Build history of the part. All positions in model axes, mm. A direction names the side the tool comes from. Round coordinates to 2 decimals unless told otherwise and drop trailing zeros. Loops run counter-clockwise (first coordinate to the right, second up) from the corner with the lowest first, then second, coordinate; pieces in that order, holes last.
from build123d import *

# Parameters (mm, degrees)
SKETCH1_R                    = 33.334829616
SKETCH1_R_2                  = 11
EXTRUDE1_DEPTH               = 10
SKETCH2_W                    = 68.7469374
SKETCH2_H                    = 68.7469374
CUT_EXTRUDE1_DEPTH           = 10
SKETCH3_R                    = 1.5
CUT_EXTRUDE2_DEPTH           = 32.563829392
SKETCH4_R                    = 2.25
CUT_EXTRUDE3_DEPTH           = 1.5
CUT_EXTRUDE3_DRAFT           = -28
CUT_EXTRUDE3_PROFILE_2_DEPTH = 1.5
CUT_EXTRUDE3_PROFILE_2_DRAFT = -28
CUT_EXTRUDE3_PROFILE_3_DEPTH = 1.5
CUT_EXTRUDE3_PROFILE_3_DRAFT = -28
CUT_EXTRUDE3_PROFILE_4_DEPTH = 1.5
CUT_EXTRUDE3_PROFILE_4_DRAFT = -28
SKETCH5_R                    = 13.5
CUT_EXTRUDE4_DEPTH           = 3


with BuildPart() as part:
    # Sketch1 → Extrude1 (new body)
    with BuildSketch(Plane(origin=(0, 0, 0), x_dir=(1, 0, 0), z_dir=(0, 1, 0))):
        with Locations(Location((0, 0, 0), (0, 0, 270))):
            Circle(SKETCH1_R)
        with Locations(Location((0, 0, 0), (0, 0, 270))):
            Circle(SKETCH1_R_2, mode=Mode.SUBTRACT)
    extrude(amount=EXTRUDE1_DEPTH)

    # Sketch2 → Cut-Extrude1 (cut)
    with BuildSketch(Plane.XZ):
        Rectangle(SKETCH2_W, SKETCH2_H)
        Polygon((16.16926222, 21.16926222), (21.16926222, 16.16926222), (21.16926222, -16.16926222), (16.16926222, -21.16926222), (-16.16926222, -21.16926222), (-21.16926222, -16.16926222), (-21.16926222, 16.16926222), (-16.16926222, 21.16926222), align=None, mode=Mode.SUBTRACT)
    extrude(amount=-CUT_EXTRUDE1_DEPTH, mode=Mode.SUBTRACT)

    # Sketch3 → Cut-Extrude2 (cut, through all)
    with BuildSketch(Plane(origin=(0, 10, 0), x_dir=(1, 0, 0), z_dir=(0, 1, 0))):
        with Locations(Location((-15.518439578, 15.481538459, 0), (0, 0, 270))):
            Circle(SKETCH3_R)
        with Locations(Location((-15.481538459, -15.518439578, 0), (0, 0, 270))):
            Circle(SKETCH3_R)
        with Locations(Location((15.481538459, 15.518439578, 0), (0, 0, 270))):
            Circle(SKETCH3_R)
        with Locations(Location((15.518439578, -15.481538459, 0), (0, 0, 270))):
            Circle(SKETCH3_R)
    extrude(amount=-CUT_EXTRUDE2_DEPTH, mode=Mode.SUBTRACT)


with BuildPart() as cut_extrude3_tool:
    # Sketch4 → Cut-Extrude3 (with draft: the straight prism first)
    with BuildSketch(Plane(origin=(0, 10, 0), x_dir=(1, 0, 0), z_dir=(0, 1, 0))):
        with Locations((-15.518439578, 15.481538459)):
            Circle(SKETCH4_R)
    extrude(amount=-CUT_EXTRUDE3_DEPTH)
    # Cut-Extrude3: the draft: its side faces are tilted about the plane it starts from
    cut_extrude3_sides = [cut_extrude3_tool.faces().sort_by_distance(p)[0] for p in [
        (-17.768439578, 9.25, -15.481538459),
    ]]
    draft(cut_extrude3_sides, Plane(origin=(0, 10, 0), x_dir=(1, 0, 0), z_dir=(0, 1, 0)), CUT_EXTRUDE3_DRAFT)


with BuildPart() as part_1:
    add(part.part)

    # Cut-Extrude3: cut by cut_extrude3_tool
    add(cut_extrude3_tool.part, mode=Mode.SUBTRACT)


with BuildPart() as cut_extrude3_profile_2_tool:
    # Sketch4 → Cut-Extrude3 profile 2 (with draft: the straight prism first)
    with BuildSketch(Plane(origin=(0, 10, 0), x_dir=(1, 0, 0), z_dir=(0, 1, 0))):
        with Locations((-15.481538459, -15.518439578)):
            Circle(SKETCH4_R)
    extrude(amount=-CUT_EXTRUDE3_PROFILE_2_DEPTH)
    # Cut-Extrude3 profile 2: the draft: its side faces are tilted about the plane it starts from
    cut_extrude3_profile_2_sides = [cut_extrude3_profile_2_tool.faces().sort_by_distance(p)[0] for p in [
        (-17.731538459, 9.25, 15.518439578),
    ]]
    draft(cut_extrude3_profile_2_sides, Plane(origin=(0, 10, 0), x_dir=(1, 0, 0), z_dir=(0, 1, 0)), CUT_EXTRUDE3_PROFILE_2_DRAFT)


with BuildPart() as part_2:
    add(part_1.part)

    # Cut-Extrude3 profile 2: cut by cut_extrude3_profile_2_tool
    add(cut_extrude3_profile_2_tool.part, mode=Mode.SUBTRACT)


with BuildPart() as cut_extrude3_profile_3_tool:
    # Sketch4 → Cut-Extrude3 profile 3 (with draft: the straight prism first)
    with BuildSketch(Plane(origin=(0, 10, 0), x_dir=(1, 0, 0), z_dir=(0, 1, 0))):
        with Locations((15.481538459, 15.518439578)):
            Circle(SKETCH4_R)
    extrude(amount=-CUT_EXTRUDE3_PROFILE_3_DEPTH)
    # Cut-Extrude3 profile 3: the draft: its side faces are tilted about the plane it starts from
    cut_extrude3_profile_3_sides = [cut_extrude3_profile_3_tool.faces().sort_by_distance(p)[0] for p in [
        (13.231538459, 9.25, -15.518439578),
    ]]
    draft(cut_extrude3_profile_3_sides, Plane(origin=(0, 10, 0), x_dir=(1, 0, 0), z_dir=(0, 1, 0)), CUT_EXTRUDE3_PROFILE_3_DRAFT)


with BuildPart() as part_3:
    add(part_2.part)

    # Cut-Extrude3 profile 3: cut by cut_extrude3_profile_3_tool
    add(cut_extrude3_profile_3_tool.part, mode=Mode.SUBTRACT)


with BuildPart() as cut_extrude3_profile_4_tool:
    # Sketch4 → Cut-Extrude3 profile 4 (with draft: the straight prism first)
    with BuildSketch(Plane(origin=(0, 10, 0), x_dir=(1, 0, 0), z_dir=(0, 1, 0))):
        with Locations((15.518439578, -15.481538459)):
            Circle(SKETCH4_R)
    extrude(amount=-CUT_EXTRUDE3_PROFILE_4_DEPTH)
    # Cut-Extrude3 profile 4: the draft: its side faces are tilted about the plane it starts from
    cut_extrude3_profile_4_sides = [cut_extrude3_profile_4_tool.faces().sort_by_distance(p)[0] for p in [
        (13.268439578, 9.25, 15.481538459),
    ]]
    draft(cut_extrude3_profile_4_sides, Plane(origin=(0, 10, 0), x_dir=(1, 0, 0), z_dir=(0, 1, 0)), CUT_EXTRUDE3_PROFILE_4_DRAFT)


with BuildPart() as part_4:
    add(part_3.part)

    # Cut-Extrude3 profile 4: cut by cut_extrude3_profile_4_tool
    add(cut_extrude3_profile_4_tool.part, mode=Mode.SUBTRACT)

    # Sketch5 → Cut-Extrude4 (cut)
    with BuildSketch(Plane(origin=(0, 10, 0), x_dir=(1, 0, 0), z_dir=(0, 1, 0))):
        with Locations(Location((0, 0, 0), (0, 0, 270))):
            Circle(SKETCH5_R)
    extrude(amount=-CUT_EXTRUDE4_DEPTH, mode=Mode.SUBTRACT)


solid = part_4.part
(1) Pull direction Z, two halves, no side cores. Call faces 3 (the face through (-10, 7, -5)), 4 (the face through (18.634, 4.93, 18.704)), 5 (the face through (0, 5, -21.169)), 6 (the face through (-21.169, 5, 0)): +Z half, -Z half, draft (parallel to the pull), parting line (faces both ways), or undercut.
Responses:
face 3: undercut
face 4: +Z half
face 5: -Z half
face 6: draft
(2) Slice it at C-C on y = 4.25. List the corners of the cut face in (x, z).
Responses:
outline: (-21.17, -16.17) - (-16.17, -21.17) - (16.17, -21.17) - (21.17, -16.17) - (21.17, 16.17) - (16.17, 21.17) - (-16.17, 21.17) - (-21.17, 16.17) - close; hole circle Ø3 at (-15.52, -15.48); hole circle Ø3 at (-15.48, 15.52); hole circle Ø22 at (0, 0); hole circle Ø3 at (15.48, -15.52); hole circle Ø3 at (15.52, 15.48)
(3) Which spindle directions (+Z, -Z, +X, -X, +Y, -Y) get a long thin tool onto all of the face, cutting with end or side? Do faces 1 (the face through (-15.45, 4.35, -16.98)), 2 (the face through (-13.18, 8.52, -2.93)). Say none if no direction does.
Responses:
face 1: +Y, -Y
face 2: +Y
(4) Pin check, flat tip, straight feed: P1, Ø3.5, axis at x = -15.48, z = 15.52, coming from the +Y side. Stop position of the tip, or through.
Responses:
P1: stops at y = 9.06
(5) Slice it at B-B on z = 0. List the corners of the cut face in (x, y).
Responses:
outline: (-21.17, 0) - (-11, 0) - (-11, 7) - (-13.5, 7) - (-13.5, 10) - (-21.17, 10) - close; (11, 0) - (21.17, 0) - (21.17, 10) - (13.5, 10) - (13.5, 7) - (11, 7) - close
(6) Slice it at A-A on x = 0. List the corners of the cut face in (y, z), plus the area to 3 significant figures.
Responses:
outline: (0, -21.17) - (10, -21.17) - (10, -13.5) - (7, -13.5) - (7, -11) - (0, -11) - close; (0, 11) - (7, 11) - (7, 13.5) - (10, 13.5) - (10, 21.17) - (0, 21.17) - close
area: 188 mm2
(7) Slice it at D-D on z = 12.5. List the corners of the cut face in (x, y).
Responses:
outline: (-21.17, 0) - (21.17, 0) - (21.17, 10) - (5.1, 10) - (5.1, 7) - (-5.1, 7) - (-5.1, 10) - (-21.17, 10) - close
(8) Probe line 1 (X direction, y = 8.5, z = 0); line 2 (Z direction, x = 0, y = 4.5); line 3 (X direction, y = 1.25, z = 15). List the from-to ranges inside material, lowest first.
Responses:
line 1: x = -21.17 to -13.5, 13.5 to 21.17
line 2: z = -21.17 to -11, 11 to 21.17
line 3: x = -21.17 to -16.89, -14.07 to 14.1, 16.94 to 21.17
